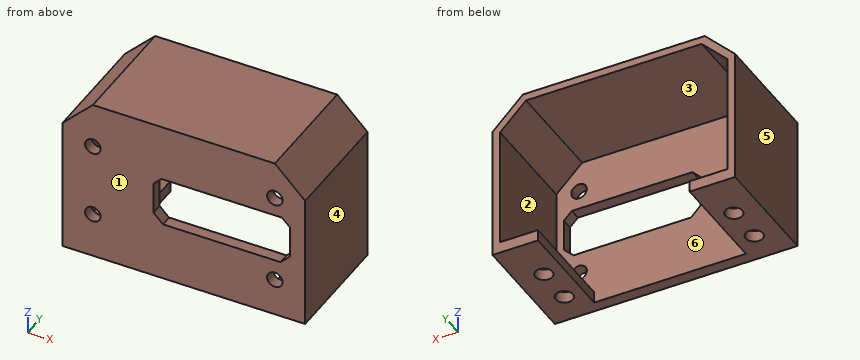
```python
from build123d import *

# Parameters (mm, degrees)
SKETCH1_W               = 12
SKETCH1_H               = 20.5
ARM_MOUNTS_DEPTH        = 3
ARM_MOUNTS_2_DEPTH      = 3
ARM_HOLES_DEPTH         = 34.735181932
ARM_HOLES_DEPTH_BACK    = 3
SKETCH2_R               = 2.25
SKETCH3_W               = 64
SKETCH3_H               = 3
BOTTOM_PLATE_DEPTH      = 28
SIDE_RIBS_DEPTH         = 2
SKETCH5_W               = 36
SKETCH5_H               = 12
CUT_EXTRUDE2_DEPTH      = 10
SKETCH6_R               = 2.05
MOUNTING_HOLES_DEPTH    = 10
CUT_EXTRUDE4_DEPTH      = 48.204343021
CUT_EXTRUDE4_DEPTH_BACK = 48.204343021
SKETCH8_W               = 64
SKETCH8_H               = 6.2
SKETCH10_W              = 64
SKETCH10_H              = 21.8
BOSS_EXTRUDE7_DEPTH     = 3
CHAMFER3_SIZE           = 5
CHAMFER4_SIZE           = 2.5
CHAMFER5_SIZE           = 8
CUT_EXTRUDE5_DEPTH      = 10
BOSS_EXTRUDE8_DEPTH     = 20.5
BOSS_EXTRUDE9_DEPTH     = 7


with BuildPart() as part:
    # Sketch1 → Arm Mounts (new body)
    with BuildSketch(Plane.XY):
        with Locations((26, 0)):
            Rectangle(SKETCH1_W, SKETCH1_H)
    extrude(amount=ARM_MOUNTS_DEPTH)


with BuildPart() as body_2:
    # Sketch1 → Arm Mounts 2 (new body)
    with BuildSketch(Plane.XY):
        with Locations((-26, 0)):
            Rectangle(SKETCH1_W, SKETCH1_H)
    extrude(amount=ARM_MOUNTS_2_DEPTH)


with BuildPart() as arm_holes_tool:
    # Sketch2 → Arm Holes (new, two sides: drawn at the far end of the back side and taken through both)
    with BuildSketch(Plane(origin=(0, 0, 3), x_dir=(-1, 0, 0), z_dir=(0, 0, -1)).offset(-ARM_HOLES_DEPTH_BACK)):
        with Locations(Location((25.05, 5, 0), (0, 0, 180))):
            Circle(SKETCH2_R)
        with Locations(Location((25.05, -5, 0), (0, 0, 180))):
            Circle(SKETCH2_R)
        with Locations(Location((-25.05, -5, 0), (0, 0, 180))):
            Circle(SKETCH2_R)
        with Locations(Location((-25.05, 5, 0), (0, 0, 180))):
            Circle(SKETCH2_R)
    extrude(amount=ARM_HOLES_DEPTH + ARM_HOLES_DEPTH_BACK)


with BuildPart() as part_1:
    add(part.part)

    # Arm Holes: cut by arm_holes_tool
    add(arm_holes_tool.part, mode=Mode.SUBTRACT)



with BuildPart() as body_2_1:
    add(body_2.part)

    # Arm Holes: cut by arm_holes_tool
    add(arm_holes_tool.part, mode=Mode.SUBTRACT)


with BuildPart() as part_2:
    add(part_1.part)

    add(body_2_1.part)  # Bottom Plate merges body 2
    # Sketch3 → Bottom Plate (add)
    with BuildSketch(Plane(origin=(0, 0, 0), x_dir=(-1, 0, 0), z_dir=(0, 0, -1))):
        with Locations((0, -11.75)):
            Rectangle(SKETCH3_W, SKETCH3_H)
    extrude(amount=-BOTTOM_PLATE_DEPTH)

    # Sketch4 → Side Ribs (add)
    with BuildSketch(Plane.ZY.offset(32)):
        Polygon((3, 10.25), (28, -10.25), (3, -10.25), align=None)
    side_ribs = extrude(amount=-SIDE_RIBS_DEPTH)

    # Rib Mirror: Side Ribs across plane
    add(side_ribs.mirror(Plane(origin=(0, 0, 0), x_dir=(0, 0, 1), z_dir=(1, 0, 0))))

    # Sketch5 → Cut-Extrude2 (cut)
    with BuildSketch(Plane(origin=(0, -10.25, 0), x_dir=(1, 0, 0), z_dir=(0, 1, 0))):
        with Locations((10, -22)):
            Rectangle(SKETCH5_W, SKETCH5_H)
    cut_extrude2 = extrude(amount=-CUT_EXTRUDE2_DEPTH, mode=Mode.SUBTRACT)

    # Sketch6 → Mounting Holes (cut)
    with BuildSketch(Plane(origin=(0, -10.25, 0), x_dir=(1, 0, 0), z_dir=(0, 1, 0))):
        with Locations(Location((-24, -12, 0), (0, 0, 270))):
            Circle(SKETCH6_R)
        with Locations(Location((24, -10, 0), (0, 0, 270))):
            Circle(SKETCH6_R)
    mounting_holes = extrude(amount=-MOUNTING_HOLES_DEPTH, mode=Mode.SUBTRACT)

    # Sketch8 → Cut-Extrude4 (cut, two sides: drawn at the far end of the back side and taken through both)
    with BuildSketch(Plane(origin=(0, -10.25, 0), x_dir=(1, 0, 0), z_dir=(0, 1, 0)).offset(-CUT_EXTRUDE4_DEPTH_BACK)):
        with Locations((0, -24.9)):
            Rectangle(SKETCH8_W, SKETCH8_H)
    extrude(amount=CUT_EXTRUDE4_DEPTH + CUT_EXTRUDE4_DEPTH_BACK, mode=Mode.SUBTRACT)

    # Sketch10 → Boss-Extrude7 (add)
    with BuildSketch(Plane(origin=(0, -10.25, 0), x_dir=(1, 0, 0), z_dir=(0, 1, 0))):
        with Locations((0, -32.7)):
            Rectangle(SKETCH10_W, SKETCH10_H)
    extrude(amount=-BOSS_EXTRUDE7_DEPTH)

    # Mirror5: Cut-Extrude2, Mounting Holes across plane
    add(cut_extrude2.mirror(Plane.XY.offset(21.8)), mode=Mode.SUBTRACT)
    add(mounting_holes.mirror(Plane.XY.offset(21.8)), mode=Mode.SUBTRACT)

    # Chamfer3
    chamfer3_edges = [part_2.edges().sort_by_distance(p)[0] for p in [
        (31, -10.25, 21.8),
        (-31, -10.25, 21.8),
    ]]
    chamfer(chamfer3_edges, length=CHAMFER3_SIZE)

    # Chamfer4
    chamfer4_edges = [part_2.edges().sort_by_distance(p)[0] for p in [
        (28, -11.75, 15.6),
        (28, -11.75, 27.6),
        (-8, -11.75, 27.6),
        (-8, -11.75, 15.6),
    ]]
    chamfer(chamfer4_edges, length=CHAMFER4_SIZE)

    # Chamfer5
    chamfer5_edges = [part_2.edges().sort_by_distance(p)[0] for p in [
        (32, -11.75, 43.6),
        (-32, -11.75, 43.6),
    ]]
    chamfer(chamfer5_edges, length=CHAMFER5_SIZE)

    # Sketch11 → Cut-Extrude5 (cut)
    with BuildSketch(Plane(origin=(0, -10.25, 0), x_dir=(1, 0, 0), z_dir=(0, 1, 0))):
        Polygon((-8, -25.1), (-8, -26.514213562), (-5.914213562, -28.6), (25.914213562, -28.6), (28, -26.514213562), (28, -25.1), align=None)
    extrude(amount=-CUT_EXTRUDE5_DEPTH, mode=Mode.SUBTRACT)

    # Sketch12 → Boss-Extrude8 (add)
    with BuildSketch(Plane(origin=(0, -10.25, 0), x_dir=(1, 0, 0), z_dir=(0, 1, 0))):
        Polygon((-32, -26.8), (-32, -3), (-30, -3), (-30, -26.8), (-30, -34.771572875), (-23.171572875, -41.6), (23.171572875, -41.6), (30, -34.771572875), (30, -26.8), (30, -3), (32, -3), (32, -26.8), (32, -35.6), (24, -43.6), (-24, -43.6), (-32, -35.6), align=None)
    extrude(amount=BOSS_EXTRUDE8_DEPTH)

    # Sketch13 → Boss-Extrude9 (add)
    with BuildSketch(Plane(origin=(0, 10.25, 0), x_dir=(1, 0, 0), z_dir=(0, 1, 0))):
        Polygon((-20, 0), (-32, 0), (-32, -35.6), (-24, -43.6), (24, -43.6), (32, -35.6), (32, 0), (20, 0), (20, -3), (30, -3), (30, -34.771572875), (23.171572875, -41.6), (-23.171572875, -41.6), (-30, -34.771572875), (-30, -3), (-20, -3), align=None)
    extrude(amount=BOSS_EXTRUDE9_DEPTH)


solid = part_2.part
```
CAD build for the part. Positions are in the model's coordinates, mm. Face numbers are marked on the shaded views. A direction names the side the tool comes from. Round coordinates to 2 decimals unless told otherwise and drop trailing zeros. Order: outer loops, then holes, each group sorted by start corner. A loop starts at its lowest first (then second) coordinate and runs counter-clockwise, first axis right, second up. Notation, with made-up numbers: (32.5, -1) - (60.5, -1) arc R29 cw to (60.5, 25) - close; hole circle Ø1 at (87.25, 67). An arc over 180 degrees is marked (long way). Answer as CSV lines item,"result". Start each with the question number.
1. Saw through at B-B, the plane y = -5. Write the cut outline in (x, z), and give its area (3 significant figures).
2. Saw through at D-D, the plane z = 37.5. Write the cut outline in (x, y).
3. Pull direction X, two halves, no side cores. Call the marked faces 3, 4, 5 and 6: +X half, -X half, draft (parallel to the pull), parting line (faces both ways), or undercut.
4. Pin check, flat tips, straight feed: pin 1 (14 mm diameter, centred on x = -10, y = 9.5, fed in from -Z); pin 2 (4 mm diameter, centred on x = 25.05, y = 5, fed in from -Z); pin 3 (21 mm diameter, centred on x = -4, z = 26, fed in from +Y). Stop position of each tip, or through.
5. Saw through at C-C, the plane x = -25.05. Write the cut outline in (y, z).
6. Saw through at A-A, the plane x = -4. Write the cut outline in (y, z).
7. Drill centre lines: L1, parallel to Y at x = 25.05, z = 1.5; L2, parallel to X at y = 8, z = 8; L3, parallel to Z at x = 21.5, y = -10. Where is each one in solid material? Low to high. Write a range as [from, to].
8. Tool access for the marked faces 1 and 2: list every direction of +Z, -Z, +X, -X, +Y, -Y with a clear straight run to the whole face (end or side of a thin tool).
Model answer:
1,outline,"(-32, 0) - (-27.3, 0) - (-27.3, 3) - (-30, 3) - (-30, 34.77) - (-23.17, 41.6) - (23.17, 41.6) - (30, 34.77) - (30, 3) - (27.3, 3) - (27.3, 0) - (32, 0) - (32, 35.6) - (24, 43.6) - (-24, 43.6) - (-32, 35.6) - close; (-22.8, 0) - (-20, 0) - (-20, 3) - (-22.8, 3) - close; (20, 0) - (22.8, 0) - (22.8, 3) - (20, 3) - close"
1,area,"310 mm²"
2,outline,"(-30.1, -13.25) - (30.1, -13.25) - (30.1, 17.25) - (27.27, 17.25) - (27.27, -10.25) - (-27.27, -10.25) - (-27.27, 17.25) - (-30.1, 17.25) - close"
3,face 3,"undercut"
3,face 4,"+X half"
3,face 5,"-X half"
3,face 6,"undercut"
4,pin 1,"stops at z = 41.6"
4,pin 2,"stops at z = 37.72"
4,pin 3,"stops at y = -10.25"
5,outline,"(-13.25, 0) - (-7.25, 0) - (-7.25, 3) - (-10.25, 3) - (-10.25, 10.24) - (-13.25, 10.24) - close; (-13.25, 13.76) - (-10.25, 13.76) - (-10.25, 29.84) - (-13.25, 29.84) - close; (-13.25, 33.36) - (-10.25, 33.36) - (-10.25, 39.72) - (17.25, 39.72) - (17.25, 42.55) - (-13.25, 42.55) - close; (-2.75, 0) - (2.75, 0) - (2.75, 3) - (-2.75, 3) - close; (7.25, 0) - (17.25, 0) - (17.25, 3) - (7.25, 3) - close"
6,outline,"(-13.25, 0) - (-10.25, 0) - (-10.25, 15.6) - (-13.25, 15.6) - close; (-13.25, 28.6) - (-10.25, 28.6) - (-10.25, 41.6) - (17.25, 41.6) - (17.25, 43.6) - (-13.25, 43.6) - close"
7,L1,"y = [-13.25, -7.25], [-2.75, 2.75], [7.25, 17.25]"
7,L2,"x = [-32, -30], [30, 32]"
7,L3,"z = [0, 3], [41.6, 43.6]"
8,face 1,"+Z, -Z, +X, -X, -Y"
8,face 2,"+Y"
